Autodesk Inventor part; units mm, degrees
ref_plane "Work Plane3" through (19.3185, -5.1764, 0) normal (-0.9659, 0.2588, 0) x (-0.2588, -0.9659, 0)
ref_plane "YZ Plane" through (0, 0, 0) normal (1, 0, 0) x (0, 1, 0)
ref_plane "XZ Plane" through (0, 0, 0) normal (0, 1, 0) x (-1, 0, 0)
sketch "Sketch1" plane through (0, 0, 0) normal (0, 0, 1) x (1, 0, 0)
  circle A0 centre (0, 0) radius 55
  circle A1 centre (0, 0) radius 50
  circle A2 centre (0, 0) radius 4
  line L0 (0, 20) -> (0, 40)
  arc A3 (0, 20) -> (-10, 17.3205) centre (0, 0) ccw
  line L1 (0, 0) -> (-10, 17.3205) construction
  line L2 (0, 0) -> (0, 20) construction
  arc A4 (0, 40) -> (-20, 34.641) centre (0, 0) ccw
  line L3 (0, 0) -> (-20, 34.641) construction
  line L4 (0, 0) -> (0, 40) construction
  line L5 (-10, 17.3205) -> (-20, 34.641)
  line L6 (-17.3205, 10) -> (-34.641, 20)
  arc A5 (-17.3205, 10) -> (-20, 0) centre (0, 0) ccw
  line L7 (0, 0) -> (-20, 0) construction
  line L8 (0, 0) -> (-17.3205, 10) construction
  arc A6 (-34.641, 20) -> (-40, 0) centre (0, 0) ccw
  line L9 (0, 0) -> (-40, 0) construction
  line L10 (0, 0) -> (-34.641, 20) construction
  line L11 (-20, 0) -> (-40, 0)
  line L12 (-17.3205, -10) -> (-34.641, -20)
  arc A7 (-17.3205, -10) -> (-10, -17.3205) centre (0, 0) ccw
  line L13 (0, 0) -> (-10, -17.3205) construction
  line L14 (0, 0) -> (-17.3205, -10) construction
  arc A8 (-34.641, -20) -> (-20, -34.641) centre (0, 0) ccw
  line L15 (0, 0) -> (-20, -34.641) construction
  line L16 (0, 0) -> (-34.641, -20) construction
  line L17 (-10, -17.3205) -> (-20, -34.641)
  line L18 (0, -20) -> (0, -40)
  arc A9 (0, -20) -> (10, -17.3205) centre (0, 0) ccw
  line L19 (0, 0) -> (10, -17.3205) construction
  line L20 (0, 0) -> (0, -20) construction
  arc A10 (0, -40) -> (20, -34.641) centre (0, 0) ccw
  line L21 (0, 0) -> (20, -34.641) construction
  line L22 (0, 0) -> (0, -40) construction
  line L23 (10, -17.3205) -> (20, -34.641)
  line L24 (17.3205, -10) -> (34.641, -20)
  arc A11 (17.3205, -10) -> (20, 0) centre (0, 0) ccw
  line L25 (0, 0) -> (20, 0) construction
  line L26 (0, 0) -> (17.3205, -10) construction
  arc A12 (34.641, -20) -> (40, 0) centre (0, 0) ccw
  line L27 (0, 0) -> (40, 0) construction
  line L28 (0, 0) -> (34.641, -20) construction
  line L29 (20, 0) -> (40, 0)
  line L30 (17.3205, 10) -> (34.641, 20)
  arc A13 (17.3205, 10) -> (10, 17.3205) centre (0, 0) ccw
  line L31 (0, 0) -> (10, 17.3205) construction
  line L32 (0, 0) -> (17.3205, 10) construction
  arc A14 (34.641, 20) -> (20, 34.641) centre (0, 0) ccw
  line L33 (0, 0) -> (20, 34.641) construction
  line L34 (0, 0) -> (34.641, 20) construction
  line L35 (10, 17.3205) -> (20, 34.641)
  point P0 (0, 10)
  point P1 (-2.5882, 9.6593)
  point P2 (-5, 8.6603)
  point P3 (-7.0711, 7.0711)
  point P4 (-8.6603, 5)
  point P5 (-9.6593, 2.5882)
  point P6 (-10, 0)
  point P7 (-9.6593, -2.5882)
  point P8 (-8.6603, -5)
  point P9 (-7.0711, -7.0711)
  point P10 (-5, -8.6603)
  point P11 (-2.5882, -9.6593)
  point P12 (0, -10)
  point P13 (2.5882, -9.6593)
  point P14 (5, -8.6603)
  point P15 (7.0711, -7.0711)
  point P16 (8.6603, -5)
  point P17 (9.6593, -2.5882)
  point P18 (10, 0)
  point P19 (9.6593, 2.5882)
  point P20 (8.6603, 5)
  point P21 (7.0711, 7.0711)
  point P22 (5, 8.6603)
  point P23 (2.5882, 9.6593)
  point P24 (10.3528, -38.637)
  point P25 (20, -34.641)
  point P26 (28.2843, -28.2843)
  point P27 (34.641, -20)
  point P28 (38.637, -10.3528)
  point P29 (40, 0)
  point P30 (38.637, 10.3528)
  point P31 (34.641, 20)
  point P32 (28.2843, 28.2843)
  point P33 (20, 34.641)
  point P34 (10.3528, 38.637)
  point P35 (0, 40)
  point P36 (-10.3528, 38.637)
  point P37 (-20, 34.641)
  point P38 (-28.2843, 28.2843)
  point P39 (-34.641, 20)
  point P40 (-38.637, 10.3528)
  point P41 (-40, 0)
  point P42 (-38.637, -10.3528)
  point P43 (-34.641, -20)
  point P44 (-28.2843, -28.2843)
  point P45 (-20, -34.641)
  point P46 (-10.3528, -38.637)
  dimension "d1" = 100
  dimension "d2" = 8
  dimension "d11" = 20
  dimension "d12" = 20
  dimension "d13" = 30
  dimension "d14" = 30
  dimension "d17" = 360
  dimension "d34" = 10
  dimension "d37" = 360
  dimension "d48" = 360
  dimension "d57" = 110
extrude "Extrusion1" add sketch "Sketch1" along normal blind 10 contours A1
extrude "Extrusion2" add sketch "Sketch1" along normal blind 5.5 contours A0
hole "Hole2" at (-2.5882, -9.6593, 0) at (-7.0711, 7.0711, 0) at (9.6593, 2.5882, 0) direction (0, 0, 1) diameter 4 end through all counterbore diameter 7 counterbore depth 4
hole "Hole3" at (28.2843, -28.2843, 0) at (-38.637, -10.3528, 0) at (10.3528, 38.637, 0) direction (0, 0, 1) diameter 4 end through all counterbore diameter 7 counterbore depth 4
chamfer "Chamfer2" distance 3.5 distance2 5 1 edges at (-55, 0, 5.5) measured on face at (-50.386, -22.0512, 3.6667)
ref_plane "Work Plane3" through (19.3185, -5.1764, 0) normal (-0.9659, 0.2588, 0) x (-0.2588, -0.9659, 0)
sketch "Sketch3" plane through (19.3185, -5.1764, 0) normal (-0.9659, 0.2588, 0) x (-0.2588, -0.9659, 0)
  point P0 (0, 0)
  point P1 (0, 5)
  dimension "d61" = 5
hole "Hole4" at (19.3185, -5.1764, 5) direction (-0.9659, 0.2588, 0) diameter 3.5 depth 20
properties part number "wheel small" material "UHMW, Black"
The listing builds one solid part. Answer for the finished solid, in the listing's coordinates (mm). A direction names the side the tool comes from. Give positions to 0.01 mm unless a question says otherwise; leave off trailing zeros. One line per item, written item: value.
1. Each of these flat-tipped pins is pushed along its axis until it touches: P1, Ø6.5, axis at x = 10.35, y = 38.64, coming from the -Z side; P2, Ø2, axis at x = 35, z = 2.5, coming from the -Y side; P3, Ø3.5, axis at x = 28.28, y = -28.28, coming from the -Z side; P4, Ø5, axis at y = -35, z = 1, coming from the +X side. Where does it stop, or does it pass through?
Found:
P1: z = 4
P2: y = -43.13
P3: through
P4: x = 44.37
2. Find the intervals of material crossed by probe 1 along X at (y, z) = (-31.5, 7.75); probe 2 along Y at (x, z) = (14, 8.75); probe 3 along X at (y, z) = (28, 4), in increasing order.
Found:
probe 1: -38.83 to -24.65, -18.19 to 0, 18.19 to 38.83
probe 2: -48 to -37.47, -24.25 to 14.28, 24.25 to 48
probe 3: -43.99 to -16.17, 0 to 16.17, 28.57 to 43.99
3. For faces 1 (the face through (-14.93, -25.86, 4.93)), 2 (the face through (-3.64, -6.32, 2.03)), determine the directions among +Z, -Z, +X, -X, +Y, -Y from which every point of the face is accessible in a straight line to the end or side of a thin tool.
Found:
face 1: +Z, -Z
face 2: -Z
4. Section A-A on y = -21.5 is taken. State how many separate pieces and enclosed holes the cut face has, plus the area to 3 significant figures.
Found:
separate pieces: 3
enclosed holes: 0
area: 607 mm^2
5. For a pull along Y with two mould halves and no side action, classify faces 3 (the face through (28.13, -31.78, 2.03)), 4 (the face through (11, -11, 0)), 5 (the face through (10.2, 35.14, 2.03)) as pulls with the +Y half, pulls with the -Y half, needs draft (parallel to the pull), parting line crosses it, or undercut.
Found:
face 3: undercut
face 4: needs draft
face 5: undercut
